Design review of the part built by this model. Coordinates are the model's own, in mm. Face numbers are marked on the shaded views. A direction names the side the tool comes from. Round coordinates to 2 decimals unless told otherwise and drop trailing zeros. Loops run counter-clockwise (first coordinate to the right, second up) from the corner with the lowest first, then second, coordinate; pieces in that order, holes last. Notation, with made-up numbers: M 25.25,45.25 L 84.25,45.25 A24 cw 84.25,66.25 Z; hole C 0,-15.5 d4. An arc over 180 degrees is marked long. One line per item, written item: value. Start each with the question number.
Item 1: Mouldability with a two-part tool opening along Z and no side actions: class the marked faces 1, 2, 3 and 4 as released by +Z, released by -Z, zero draft, split by the parting line, or undercut.
Item 2: We need section A-A (y = -11). Write out the cut boundary in (x, z).
Item 3: We need section B-B (y = -27). Write out the cut boundary in (x, z).
Item 4: Clearance check with flat-ended pins moving along their axes: pin 1 (3 mm diameter, centred on x = 17.5, z = 1, fed in from +Y); pin 2 (3 mm diameter, centred on x = -16.1, z = -16.1, fed in from +Y); pin 3 (4 mm diameter, centred on x = 14.5, y = -18, fed in from -Z); pin 4 (12 mm diameter, centred on x = -10, z = -12, fed in from +Y). State where each tip first meets the part, or that it passes through.
Item 5: For the marked faces 5, 6 and 7, list the 3-axis set-ups (+Z, -Z, +X, -X, +Y, -Y) from which the entire face can be reached by the end or side of a thin tool; tool diameter is ignored.
Item 6: We need section C-C (z = 16.1). State how many separate pieces and enclosed holes the cut face has, then the cut area to 3 significant figures.
Item 7: For line 1 along Z through (x, y) = (-16.1, -9.7); line 2 along X through (y, z) = (-3, -10); line 3 along X through (y, z) = (-11, -16), list the stretches that pass through material, from the lowest coordinate up.
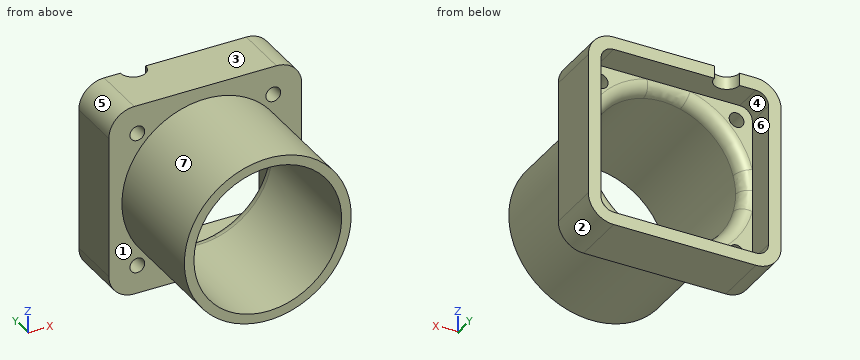
from build123d import *

# Parameters (mm, degrees)
F1_DEPTH  = 40
F2_R      = 1.75
F2_R_2    = 17.5
F3_DEPTH  = 40
F5_DEPTH  = 7
F6_R      = 29.829499
F6_R_2    = 19.768838
F7_DEPTH  = 27
F8_R      = 3
F9_R      = 3
F10_DEPTH = 3


with BuildPart() as f1:
    # F0 (on Front) → F1 (new body)
    with BuildSketch(Plane.XZ):
        with BuildLine():
            Line((16.85, 22.85), (-16.85, 22.85))
            ThreePointArc((-16.85, 22.85), (-21.092641, 21.092641), (-22.85, 16.85))
            Line((-22.85, 16.85), (-22.85, -16.85))
            ThreePointArc((-22.85, -16.85), (-21.092641, -21.092641), (-16.85, -22.85))
            Line((-16.85, -22.85), (16.85, -22.85))
            ThreePointArc((16.85, -22.85), (21.092641, -21.092641), (22.85, -16.85))
            Line((22.85, -16.85), (22.85, 16.85))
            ThreePointArc((22.85, 16.85), (21.092641, 21.092641), (16.85, 22.85))
        make_face()
        with BuildLine():
            ThreePointArc((-19.85, 16.85), (-18.97132, 18.97132), (-16.85, 19.85))
            Line((-16.85, 19.85), (16.85, 19.85))
            ThreePointArc((16.85, 19.85), (18.97132, 18.97132), (19.85, 16.85))
            Line((19.85, 16.85), (19.85, -16.85))
            ThreePointArc((19.85, -16.85), (18.97132, -18.97132), (16.85, -19.85))
            Line((16.85, -19.85), (-16.85, -19.85))
            ThreePointArc((-16.85, -19.85), (-18.97132, -18.97132), (-19.85, -16.85))
            Line((-19.85, -16.85), (-19.85, 16.85))
        make_face(mode=Mode.SUBTRACT)
    extrude(amount=F1_DEPTH)

    # F2 (on face) → F3 (join, through all)
    with BuildSketch(Plane(origin=(0, 0, 0), x_dir=(-1, 0, 0), z_dir=(0, 1, 0))):
        with BuildLine():
            ThreePointArc((-16.85, 19.85), (-18.97132, 18.97132), (-19.85, 16.85))
            Line((-19.85, 16.85), (-19.85, -16.85))
            ThreePointArc((-19.85, -16.85), (-18.97132, -18.97132), (-16.85, -19.85))
            Line((-16.85, -19.85), (16.85, -19.85))
            ThreePointArc((16.85, -19.85), (18.97132, -18.97132), (19.85, -16.85))
            Line((19.85, -16.85), (19.85, 16.85))
            ThreePointArc((19.85, 16.85), (18.97132, 18.97132), (16.85, 19.85))
            Line((16.85, 19.85), (-16.85, 19.85))
        make_face()
        with Locations((-16.1, -16.1)):
            Circle(F2_R, mode=Mode.SUBTRACT)
        with Locations((16.1, -16.1)):
            Circle(F2_R, mode=Mode.SUBTRACT)
        with Locations((-16.1, 16.1)):
            Circle(F2_R, mode=Mode.SUBTRACT)
        Circle(F2_R_2, mode=Mode.SUBTRACT)
        with Locations((16.1, 16.1)):
            Circle(F2_R, mode=Mode.SUBTRACT)
    extrude(amount=-F3_DEPTH)

    # F4 (on face) → F5 (cut)
    with BuildSketch(Plane(origin=(0, 0, 0), x_dir=(-1, 0, 0), z_dir=(0, 1, 0))):
        with BuildLine():
            Line((19.85, -16.85), (19.85, 16.85))
            ThreePointArc((19.85, 16.85), (18.97132, 18.97132), (16.85, 19.85))
            Line((16.85, 19.85), (-16.85, 19.85))
            ThreePointArc((-16.85, 19.85), (-18.97132, 18.97132), (-19.85, 16.85))
            Line((-19.85, 16.85), (-19.85, -16.85))
            ThreePointArc((-19.85, -16.85), (-18.97132, -18.97132), (-16.85, -19.85))
            Line((-16.85, -19.85), (16.85, -19.85))
            ThreePointArc((16.85, -19.85), (18.97132, -18.97132), (19.85, -16.85))
        make_face()
    extrude(amount=-F5_DEPTH, mode=Mode.SUBTRACT)

    # F6 (on face) → F7 (cut)
    with BuildSketch(Plane.XZ.offset(40)):
        Circle(F6_R)
        Circle(F6_R_2, mode=Mode.SUBTRACT)
    extrude(amount=-F7_DEPTH, mode=Mode.SUBTRACT)

    # F8
    f8_edges = [f1.edges().sort_by_distance(p)[0] for p in [
        (17.5, -7, 0),
    ]]
    fillet(f8_edges, radius=F8_R)

    # F9 (on face) → F10 (cut, through all)
    with BuildSketch(Plane.XY.offset(22.85)):
        with Locations((-10, 0)):
            Circle(F9_R)
    extrude(amount=-F10_DEPTH, mode=Mode.SUBTRACT)


solid = f1.part
A:
1. face 1: zero draft
1. face 2: released by -Z
1. face 3: released by +Z
1. face 4: undercut
2. outline: M -22.85,-16.85 A6 ccw -16.85,-22.85 L 16.85,-22.85 A6 ccw 22.85,-16.85 L 22.85,16.85 A6 ccw 16.85,22.85 L -16.85,22.85 A6 ccw -22.85,16.85 Z; hole C -16.1,-16.1 d3.5; hole C -16.1,16.1 d3.5; hole C 0,0 d35; hole C 16.1,-16.1 d3.5; hole C 16.1,16.1 d3.5
3. outline: C 0,0 d39.54; hole C 0,0 d35
4. pin 1: y = -7.32
4. pin 2: through
4. pin 3: z = -15.32
4. pin 4: y = -7
5. face 5: +Z, -X, +Y, -Y
5. face 6: +Y
5. face 7: -Y
6. separate pieces: 4
6. enclosed holes: 0
6. area: 432 mm2
7. line 1: -22.85 to -17.85, -14.35 to -6.9, 6.9 to 14.35, 17.85 to 22.85
7. line 2: -22.85 to -19.85, 19.85 to 22.85
7. line 3: -22.85 to -17.85, -14.35 to -7.09, 7.09 to 14.35, 17.85 to 22.85
